```python
from build123d import *

# Parameters (mm, degrees)
F0_W      = 15
F0_H      = 15
F1_DEPTH  = 13
F2_R      = 7
F3_DEPTH  = 5
F5_DEPTH  = 12.5
F6_R      = 7
F7_DEPTH  = 7.5
F9_DEPTH  = 8
F10_R     = 5
F11_DEPTH = 13
F16_R     = 1.5
F17_DEPTH = 25


with BuildPart() as f1:
    # F0 (on Top) → F1 (new body, symmetric)
    with BuildSketch(Plane.XY):
        Rectangle(F0_W, F0_H)
    extrude(amount=F1_DEPTH, both=True)

    # F2 (on face) → F3 (join)
    with BuildSketch(Plane(origin=(0, 0, -13), x_dir=(1, 0, 0), z_dir=(0, 0, -1))):
        Circle(F2_R)
    extrude(amount=F3_DEPTH)

    # F4 (on face) → F5 (join)
    with BuildSketch(Plane(origin=(0, 0, -18), x_dir=(1, 0, 0), z_dir=(0, 0, -1))):
        with BuildLine():
            Line((-4.8989794856, -5), (4.8989794856, -5))
            ThreePointArc((4.8989794856, -5), (4.9497474683, -4.9497474683), (5, -4.8989794856))
            Line((5, -4.8989794856), (5, 4.8989794856))
            ThreePointArc((5, 4.8989794856), (4.9497474683, 4.9497474683), (4.8989794856, 5))
            Line((4.8989794856, 5), (-4.8989794856, 5))
            ThreePointArc((-4.8989794856, 5), (-4.9497474683, 4.9497474683), (-5, 4.8989794856))
            Line((-5, 4.8989794856), (-5, -4.8989794856))
            ThreePointArc((-5, -4.8989794856), (-4.9497474683, -4.9497474683), (-4.8989794856, -5))
        make_face()
    extrude(amount=F5_DEPTH)

    # F6 (on face) → F7 (join)
    with BuildSketch(Plane.XY.offset(13)):
        Circle(F6_R)
    extrude(amount=F7_DEPTH)

    # F8 (on face) → F9 (join)
    with BuildSketch(Plane.XY.offset(20.5)):
        with BuildLine():
            Line((-4.8989794856, -5), (4.8989794856, -5))
            ThreePointArc((4.8989794856, -5), (4.9497474683, -4.9497474683), (5, -4.8989794856))
            Line((5, -4.8989794856), (5, 4.8989794856))
            ThreePointArc((5, 4.8989794856), (4.9497474683, 4.9497474683), (4.8989794856, 5))
            Line((4.8989794856, 5), (-4.8989794856, 5))
            ThreePointArc((-4.8989794856, 5), (-4.9497474683, 4.9497474683), (-5, 4.8989794856))
            Line((-5, 4.8989794856), (-5, -4.8989794856))
            ThreePointArc((-5, -4.8989794856), (-4.9497474683, -4.9497474683), (-4.8989794856, -5))
        make_face()
    extrude(amount=F9_DEPTH)

    # F10 (on face) → F11 (join)
    with BuildSketch(Plane.XY.offset(28.5)):
        Circle(F10_R)
    extrude(amount=F11_DEPTH)

    # F12 (on Right) → F13 (revolve, cut)
    with BuildSketch(Plane.YZ):
        with BuildLine():
            Line((5, 28.5), (5, 29.2546096917))
            ThreePointArc((5, 29.2546096917), (4.6226951542, 28.8773048458), (5, 28.5))
        make_face()
    revolve(axis=Axis((0, 0, 28.5), (0, 0, -1)), mode=Mode.SUBTRACT)

    # F14 (on Front) → F15 (revolve)
    with BuildSketch(Plane.XZ):
        with BuildLine():
            Line((0, 41.5), (5, 41.5))
            ThreePointArc((5, 41.5), (2.6124860802, 42.6291713066), (0, 43.0166852265))
            Line((0, 43.0166852265), (0, 41.5))
        make_face()
    revolve(axis=Axis((0, 0, 41.5), (0, 0, 1)))

    # F16 (on face) → F17 (cut)
    with BuildSketch(Plane.YZ.offset(7.5)):
        with Locations((0, 7)):
            Circle(F16_R)
    extrude(amount=-F17_DEPTH, mode=Mode.SUBTRACT)


solid = f1.part
```
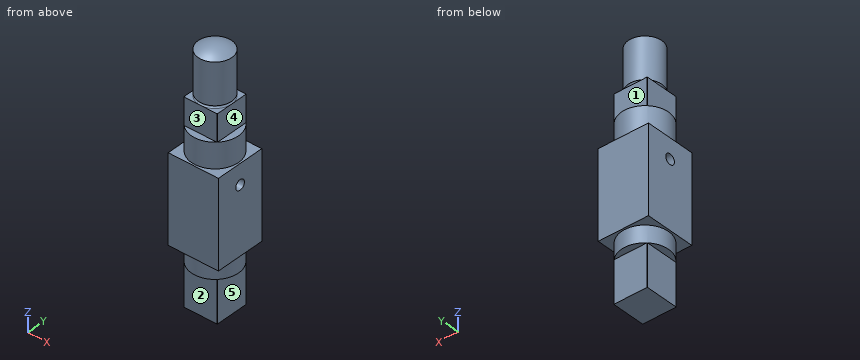
Geometry check sheet. Reference: the model listing, model coordinates, mm. Face numbers are marked on the shaded views. A direction names the side the tool comes from. Coordinates: 2 decimals unless noted, no trailing zeros. Write each loop counter-clockwise with the first axis right and the second up, starting at its lowest first coordinate (ties: lowest second). Pieces come first, ordered by that corner, then holes. Notation, with made-up numbers: M 31.25,-38 L 87.25,-38 A12 cw 87.25,-22 Z; hole C 19.25,40.25 d1. An arc over 180 degrees is marked long. Answer as a JSON object with one key per item and string values.
1. Section check A-A, the plane z = 7. Enter the section's corners in (x, y).
Answers below:
{"outline": "M -7.5,-7.5 L 7.5,-7.5 L 7.5,-1.5 L -7.5,-1.5 Z; M -7.5,1.5 L 7.5,1.5 L 7.5,7.5 L -7.5,7.5 Z"}
2. Section check C-C, the plane y = 6.25. Enter the section's corners in (x, z).
Answers below:
{"outline": "M -7.5,-13 L -3.15,-13 L -3.15,-18 L 3.15,-18 L 3.15,-13 L 7.5,-13 L 7.5,13 L 3.15,13 L 3.15,20.5 L -3.15,20.5 L -3.15,13 L -7.5,13 Z"}
3. Tool access check on the marked faces 1, 2, 3, 4 and 5. Record the directions out of +Z, -Z, +X, -X, +Y, -Y that give a thin tool (end or side, any length) a straight path to the whole face; none if there is none.
Answers below:
{"face 1": "+Z, +X, -X, +Y", "face 2": "-Z, +X, -X, -Y", "face 3": "+Z, +X, -X, -Y", "face 4": "+Z, +X, +Y, -Y", "face 5": "-Z, +X, +Y, -Y"}
4. Go/stop test with flat-tipped pins: pin 1 Ø2 at (y, z) = (1.5, 25) entering from -X; pin 2 Ø5 at (x, z) = (1, -24) entering from +Y; pin 3 Ø1.6 at (x, y) = (-2, 6.5) entering from +Z. Record where each tip stops, or that it passes through.
Answers below:
{"pin 1": "stops at x = -5", "pin 2": "stops at y = 5", "pin 3": "stops at z = 20.5"}
5. Section check D-D, the plane z = 35.5. Enter the section's corners in (x, y), plus the area to 3 significant figures.
Answers below:
{"outline": "C 0,0 d10", "area": "78.5 mm²"}
6. Scan lines: L1, parallel to Z at x = -5.5, y = 0; L2, parallel to X at y = -2.5, z = 21; L3, parallel to Z at x = 6, y = -0.75. Record each from-to range of solid material in increasing order.
Answers below:
{"L1": "z = -18 to 5.5, 8.5 to 20.5", "L2": "x = -5 to 5", "L3": "z = -18 to 5.7, 8.3 to 20.5"}
7. Section check B-B, the plane z = -19. Enter the section's corners in (x, y).
Answers below:
{"outline": "M -5,-4.9 A7 ccw -4.9,-5 L 4.9,-5 A7 ccw 5,-4.9 L 5,4.9 A7 ccw 4.9,5 L -4.9,5 A7 ccw -5,4.9 Z"}
